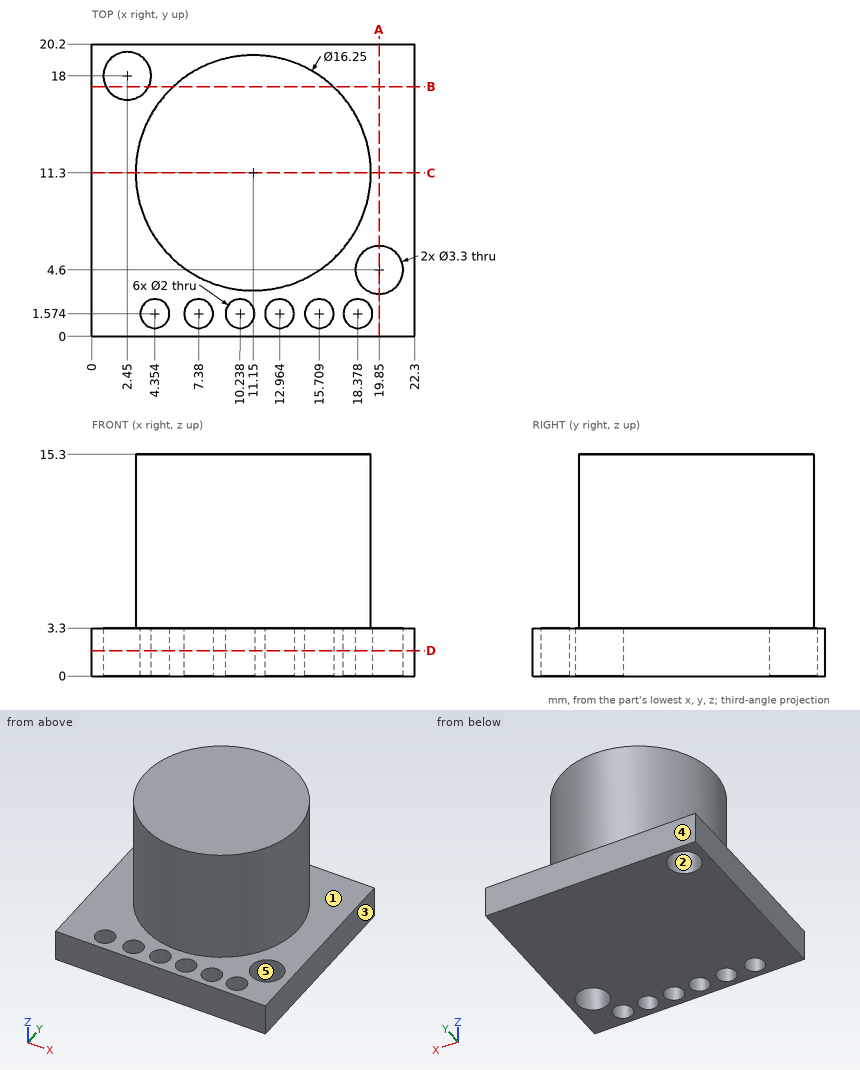
The drawing under review shows one solid part. Ordinate dimensions are in mm from its lowest x, y, z. A direction names the side the tool comes from. Coordinates: 2 decimals unless noted, no trailing zeros. Loops run counter-clockwise (first coordinate to the right, second up) from the corner with the lowest first, then second, coordinate; pieces in that order, holes last.
Item 1: Draft analysis for pull direction Y (two halves, no side actions). For the marked faces 3, 4 and 5, state which applies: pulls with the +Y half, pulls with the -Y half, needs draft (parallel to the pull), parting line crosses it, or undercut.
Completed:
face 3: needs draft
face 4: pulls with the +Y half
face 5: undercut
Item 2: Clearance check with flat-ended pins moving along their axes: pin 1 (5 mm diameter, centred on x = 4, z = 7, fed in from -Y); pin 2 (6 mm diameter, centred on x = 15, z = 13.5, fed in from +Y); pin 3 (4 mm diameter, centred on y = 18, z = 11.5, fed in from +X). State where each tip first meets the part, or that it passes through.
Completed:
pin 1: stops at y = 4.64
pin 2: stops at y = 19.38
pin 3: stops at x = 17.78
Item 3: Wall thickness on L1, parallel to Y at x = 2.45, z = 2.6; L2, parallel to Z at x = 16.25, y = 19.25; L3, parallel to X at y = 11, z = 8.5: over which ranges is each line inside the solid? List them lowest first.
Completed:
L1: y = 0 to 16.35, 19.65 to 20.2
L2: z = 0 to 3.3
L3: x = 3.03 to 19.27
Item 4: Add section C-C (y = 11.3). Write out the cut boundary in (x, z) (1 decimal), and give its area (3 significant figures).
Completed:
outline: (0, 0) - (22.3, 0) - (22.3, 3.3) - (19.3, 3.3) - (19.3, 15.3) - (3, 15.3) - (3, 3.3) - (0, 3.3) - close
area: 269 mm2
Item 5: Add section D-D (z = 1.75). Give the number of separate pieces and of enclosed holes in the cut face.
Completed:
separate pieces: 1
enclosed holes: 8
Item 6: Add section B-B (y = 17.25). Write out the cut boundary in (x, z), and give its area (3 significant figures).
Completed:
outline: (0, 0) - (0.98, 0) - (0.98, 3.3) - (0, 3.3) - close; (3.92, 0) - (22.3, 0) - (22.3, 3.3) - (16.68, 3.3) - (16.68, 15.3) - (5.62, 15.3) - (5.62, 3.3) - (3.92, 3.3) - close
area: 197 mm2
Item 7: For the marked faces 1 and 2, list the 3-axis set-ups (+Z, -Z, +X, -X, +Y, -Y) from which the entire face can be reached by the end or side of a thin tool; tool diameter is ignored.
Completed:
face 1: +Z
face 2: +Z, -Z
Item 8: Add section A-A (x = 19.85). Write out the cut boundary in (y, z).
Completed:
outline: (0, 0) - (2.95, 0) - (2.95, 3.3) - (0, 3.3) - close; (6.25, 0) - (20.2, 0) - (20.2, 3.3) - (6.25, 3.3) - close
